Source: CAD feature listing. Evaluate the final solid. Frame: model axes, mm. Face numbers are marked on the shaded views. A direction names the side the tool comes from. Give positions to 0.01 mm unless a question says otherwise; leave off trailing zeros. Loops run counter-clockwise (first coordinate to the right, second up) from the corner with the lowest first, then second, coordinate; pieces in that order, holes last.
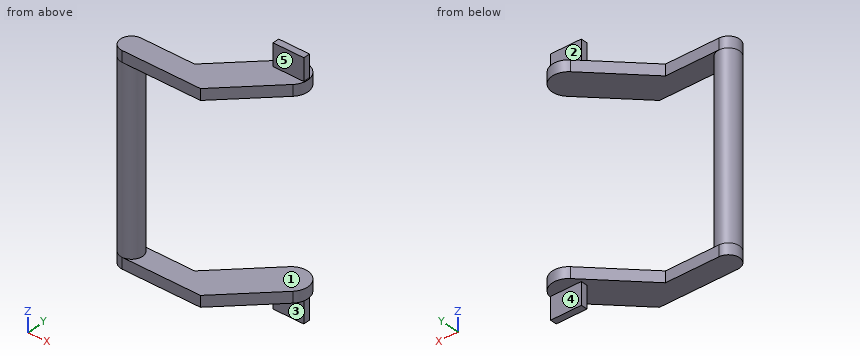
```python
from build123d import *

# Parameters (mm, degrees)
EXTRUDE_1_DEPTH        = 41
EXTRUDE_1_DEPTH_BACK   = 41
SKETCH_1_R             = 5
EXTRUDE_2_DEPTH        = 5
FILLET_1_R             = 7.5
FILLET_1_OF_MIRROR_1_R = 7.5
SKETCH_3_W             = 14
SKETCH_3_H             = 3
EXTRUDE_3_DEPTH        = 10


with BuildPart() as part:
    # 草图1 → 凸台-拉伸1 (new, two sides: drawn at the far end of the back side and taken through both)
    with BuildSketch(Plane.XY.offset(-EXTRUDE_1_DEPTH_BACK)):
        Circle(SKETCH_1_R)
    extrude(amount=EXTRUDE_1_DEPTH + EXTRUDE_1_DEPTH_BACK)

    # 草图2 → 凸台-拉伸2 (add)
    with BuildSketch(Plane.XY.offset(41)):
        with BuildLine():
            Line((0, 5), (24.393398282, 5))
            Line((24.393398282, 5), (52.980970389, 33.587572106))
            Line((52.980970389, 33.587572106), (63.587572106, 22.980970389))
            Line((63.587572106, 22.980970389), (35.606601718, -5))
            Line((35.606601718, -5), (0, -5))
            ThreePointArc((0, -5), (-5, 0), (0, 5))
        make_face()
    extrude_2 = extrude(amount=EXTRUDE_2_DEPTH)

    # 圆角1
    fillet_1_edges = [part.edges().sort_by_distance(p)[0] for p in [
        (63.587572106, 22.980970389, 43.5),
        (52.980970389, 33.587572106, 43.5),
    ]]
    fillet(fillet_1_edges, radius=FILLET_1_R - 0.0001)  # a hair under: the kernel refuses the full size

    # 镜向1: 凸台-拉伸2 across plane
    add(extrude_2.mirror(Plane.XY))

    # 圆角1 of 镜向1
    fillet_1_of_mirror_1_edges = [part.edges().sort_by_distance(p)[0] for p in [
        (63.587572106, 22.980970389, -43.5),
        (52.980970389, 33.587572106, -43.5),
    ]]
    fillet(fillet_1_of_mirror_1_edges, radius=FILLET_1_OF_MIRROR_1_R - 0.0001)  # a hair under: the kernel refuses the full size

    # 草图3 → 凸台-拉伸3 (add)
    with BuildSketch(Plane.XY.offset(46)):
        with Locations((52.980970389, 22.980970389)):
            Rectangle(SKETCH_3_W, SKETCH_3_H)
    extrude_3 = extrude(amount=EXTRUDE_3_DEPTH)

    # 镜向2: 凸台-拉伸3 across plane
    add(extrude_3.mirror(Plane.XY))


solid = part.part
```
(1) Section C-C, the plane y = 2.5. Return the cut outline in (x, z).
A:
outline: (-4.33, -46) - (43.11, -46) - (43.11, -41) - (4.33, -41) - (4.33, 41) - (43.11, 41) - (43.11, 46) - (-4.33, 46) - close
(2) Section B-B, the plane y = 26. Return the cut outline in (x, z).
A:
outline: (45.39, -46) - (59.85, -46) - (59.85, -41) - (45.39, -41) - close; (45.39, 41) - (59.85, 41) - (59.85, 46) - (45.39, 46) - close
(3) Section D-D, the plane z = -15. Return the cut outline in (x, y), then the cut area to 3 significant figures.
A:
outline: circle Ø10 at (0, 0)
area: 78.5 mm2
(4) Section A-A, the plane x = 19. Return the cut outline in (y, z), then the cut area to 3 significant figures.
A:
outline: (-5, -46) - (5, -46) - (5, -41) - (-5, -41) - close; (-5, 41) - (5, 41) - (5, 46) - (-5, 46) - close
area: 100 mm2
(5) Reachability of the marked faces 3, 4 and 5 from +Z, -Z, +X, -X, +Y, -Y: full face, straight path, thin tool, end or side. Return the list, or none.
A:
face 3: -Z, +X, -X, -Y
face 4: -Z, +X, -X, +Y
face 5: +Z, +X, -X, -Y
(6) First-contact query: pin 1 (1.5 mm diameter, centred on x = 11, z = -44.5, fed in from +Y); pin 2 (3 mm diameter, centred on x = 56, z = 51.5, fed in from -Y); pin 3 (5 mm diameter, centred on x = 50, z = -53, fed in from +Y); pin 4 (12 mm diameter, centred on y = 23, z = -31.5, fed in from -X). Flat tips, straight axial feed; report the tip coordinate or a pass-through.
A:
pin 1: stops at y = 5
pin 2: stops at y = 21.48
pin 3: stops at y = 24.48
pin 4: passes through
(7) Ray query, line 1 along Z through (x, y) = (46.5, 23.5); line 2 along Z through (x, y) = (4, 4); line 3 along X through (y, z) = (-3, 18). Return the intervals inside material, ascending.
A:
line 1: z = -56 to -41, 41 to 56
line 2: z = -46 to -41, 41 to 46
line 3: x = -4 to 4
(8) Mould query, pull axis Z, two halves, no side actions, for the marked faces 1 and 2. Classes: pulls with the +Z half, pulls with the -Z half, needs draft (parallel to the pull), parting line crosses it, or undercut.
A:
face 1: undercut
face 2: needs draft
